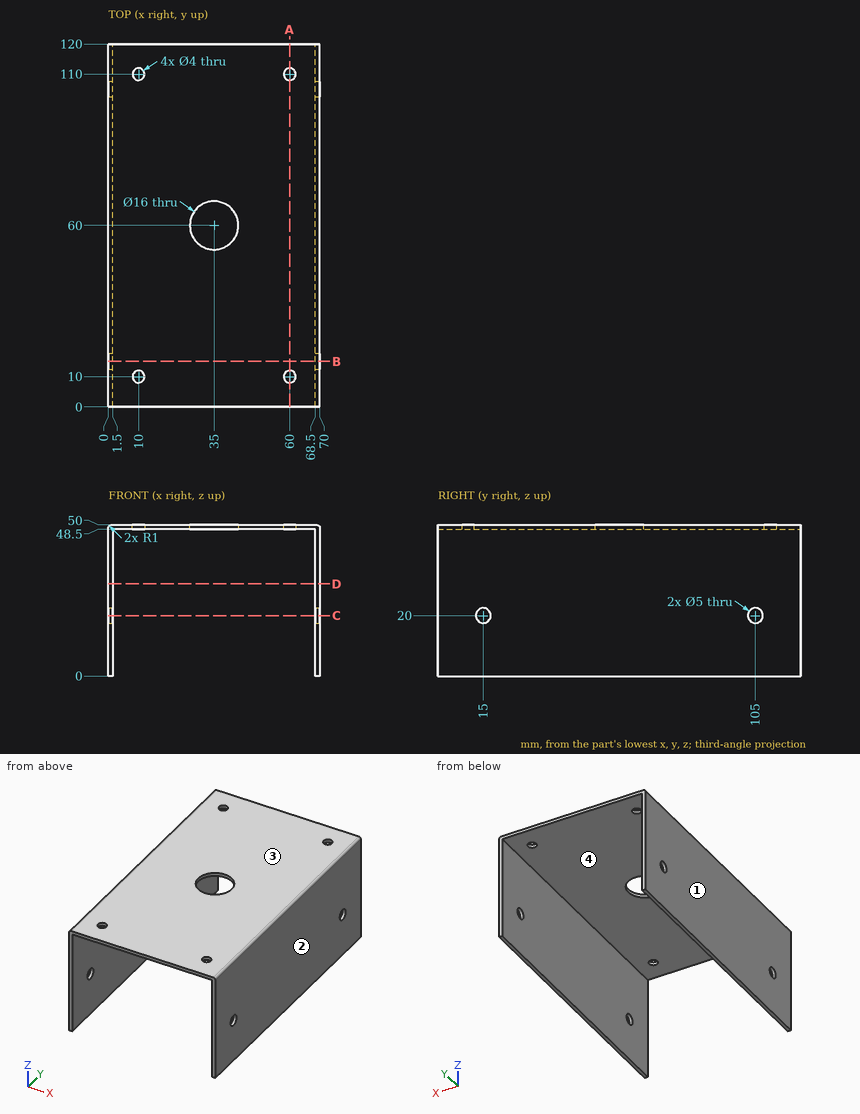
Source: three-view drawing plus pictorial views. Frame: mm from the lowest corner of the part. Give positions to 0.01 mm unless a question says otherwise; leave off trailing zeros. Loops run counter-clockwise (first coordinate to the right, second up) from the corner with the lowest first, then second, coordinate; pieces in that order, holes last.
1) Section query B-B on y = 15. Return the cut outline in (x, z), and give its area (3 significant figures).
A:
outline: (0, 0) - (1.5, 0) - (1.5, 17.5) - (0, 17.5) - close; (0, 22.5) - (1.5, 22.5) - (1.5, 48.5) - (68.5, 48.5) - (68.5, 22.5) - (70, 22.5) - (70, 49) arc R1 ccw to (69, 50) - (1, 50) arc R1 ccw to (0, 49) - close; (68.5, 0) - (70, 0) - (70, 17.5) - (68.5, 17.5) - close
area: 235 mm2
2) Section query C-C on z = 20. Return the cut outline in (x, y).
A:
outline: (0, 0) - (1.5, 0) - (1.5, 12.5) - (0, 12.5) - close; (0, 17.5) - (1.5, 17.5) - (1.5, 102.5) - (0, 102.5) - close; (0, 107.5) - (1.5, 107.5) - (1.5, 120) - (0, 120) - close; (68.5, 0) - (70, 0) - (70, 12.5) - (68.5, 12.5) - close; (68.5, 17.5) - (70, 17.5) - (70, 102.5) - (68.5, 102.5) - close; (68.5, 107.5) - (70, 107.5) - (70, 120) - (68.5, 120) - close
3) Mould query, pull axis X, two halves, no side actions, for the marked faces 1, 2, 3 and 4. Classes: released by +X, released by -X, zero draft, split by the parting line, or undercut.
A:
face 1: released by -X
face 2: released by +X
face 3: zero draft
face 4: undercut
4) Section query A-A on x = 60. Return the cut outline in (y, z).
A:
outline: (0, 48.5) - (8, 48.5) - (8, 50) - (0, 50) - close; (12, 48.5) - (108, 48.5) - (108, 50) - (12, 50) - close; (112, 48.5) - (120, 48.5) - (120, 50) - (112, 50) - close
5) Line query: L1, parallel to Y at x = 10, z = 49.5; L2, parallel to X at y = 11.5, z = 39.5; L3, parallel to Z at x = 69, y = 15. Output: solid intervals per line, ascending.
A:
L1: y = 0 to 8, 12 to 108, 112 to 120
L2: x = 0 to 1.5, 68.5 to 70
L3: z = 0 to 17.5, 22.5 to 50
6) Contact query for flat-ended pins moving along their axis: pin 1 (12 mm diameter, centred on x = 56.5, y = 35, fed in from -Z); pin 2 (4.5 mm diameter, centred on y = 15, z = 20, fed in from -X). Output: stop coordinate, or through.
A:
pin 1: stops at z = 48.5
pin 2: passes through
7) Section query D-D on z = 30.5. Return the cut outline in (x, y), and give its area (3 significant figures).
A:
outline: (0, 0) - (1.5, 0) - (1.5, 120) - (0, 120) - close; (68.5, 0) - (70, 0) - (70, 120) - (68.5, 120) - close
area: 360 mm2
